For this review, take the finished solid that the model builds, in its own axes (mm). Face numbers are marked on the shaded views. A direction names the side the tool comes from. Round coordinates to 2 decimals unless told otherwise and drop trailing zeros. Write each loop counter-clockwise with the first axis right and the second up, starting at its lowest first coordinate (ties: lowest second). Pieces come first, ordered by that corner, then holes. Notation, with made-up numbers: (23.25, 4.25) -> (61.25, 4.25) arc R34 ccw to (61.25, 41.25) -> close; hole circle Ø7 at (-18, 88). An arc over 180 degrees is marked (long way). Write each question's results on one line, items separated by ' | '. Start each with the question number.
Item 1: Add section D-D (z = 4.5). State the section outline as (x, y) points.
Item 2: Add section C-C (z = 0.75). State the section outline as (x, y) points, plus the area to 3 significant figures.
Item 3: Add section B-B (y = -2.5). State the section outline as (x, z) points.
Item 4: Clearance check with flat-ended pins moving along their axes: pin 1 (0.5 mm diameter, centred on y = -4.5, z = 2.5, fed in from +X); pin 2 (3 mm diameter, centred on x = -3, y = -2, fed in from -Z); pin 3 (3 mm diameter, centred on x = -3.5, y = -3.5, fed in from +Z). State where each tip first meets the part, or that it passes through.
Item 5: The part is to be moulded in two halves that separate along X. For the marked faces 5, 6 and 7, say which applies: +X half, -X half, draft (parallel to the pull), parting line (faces both ways), or undercut.
Item 6: To check wall thickness, follow line 1 along X through (y, z) = (-3, 2.5); line 2 along Y through (x, z) = (19.5, 1); line 3 along X through (y, z) = (-2.5, 3). State the ranges of each line that lie inside material, in increasing order.
Item 7: Add section A-A (x = -4). State the section outline as (y, z) points, plus the area to 3 significant figures.
Item 8: Tool access review of the marked faces 1, 2, 3 and 4: name each direction out of +Z, -Z, +X, -X, +Y, -Y from which nothing blocks a thin tool from reaching the whole face with its end or side.
from build123d import *

# Parameters (mm, degrees)
F1_DEPTH = 6
F2_R     = 1.5
F3_DEPTH = 1.5
F4_R     = 1.5
F4_W     = 1.5
F4_H     = 6
F5_DEPTH = 1.5


with BuildPart() as f1:
    # F0 (on Front) → F1 (new body)
    with BuildSketch(Plane.XZ):
        with BuildLine():
            Line((15, 3), (15, 0))
            Line((15, 0), (16.5, 0))
            Line((16.5, 0), (16.5, 3))
            ThreePointArc((16.5, 3), (15.474874, 5.474874), (13, 6.5))
            Line((13, 6.5), (2, 6.5))
            ThreePointArc((2, 6.5), (-0.474874, 5.474874), (-1.5, 3))
            Line((-1.5, 3), (-1.5, 2))
            Line((-1.5, 2), (0, 2))
            Line((0, 2), (0, 3))
            ThreePointArc((0, 3), (0.585786, 4.414214), (2, 5))
            Line((2, 5), (13, 5))
            ThreePointArc((13, 5), (14.414214, 4.414214), (15, 3))
        make_face()
    extrude(amount=F1_DEPTH)

    # F2 (on Top) → F3 (join)
    with BuildSketch(Plane.XY):
        with BuildLine():
            Line((16.5, 0), (16.5, -6))
            Line((16.5, -6), (19.5, -6))
            ThreePointArc((19.5, -6), (21.62132, -5.12132), (22.5, -3))
            ThreePointArc((22.5, -3), (21.62132, -0.87868), (19.5, 0))
            Line((19.5, 0), (16.5, 0))
        make_face()
        with Locations((19.5, -3)):
            Circle(F2_R, mode=Mode.SUBTRACT)
    extrude(amount=F3_DEPTH)

    # F4 (on face) → F5 (join)
    with BuildSketch(Plane(origin=(0, 0, 2), x_dir=(1, 0, 0), z_dir=(0, 0, -1))):
        with BuildLine():
            Line((-1.5, 6), (-4.5, 6))
            ThreePointArc((-4.5, 6), (-6.62132, 5.12132), (-7.5, 3))
            ThreePointArc((-7.5, 3), (-6.62132, 0.87868), (-4.5, 0))
            Line((-4.5, 0), (-1.5, 0))
            Line((-1.5, 0), (-1.5, 6))
        make_face()
        with Locations((-4.5, 3)):
            Circle(F4_R, mode=Mode.SUBTRACT)
        with Locations((-0.75, 3)):
            Rectangle(F4_W, F4_H)
    extrude(amount=-F5_DEPTH)


solid = f1.part
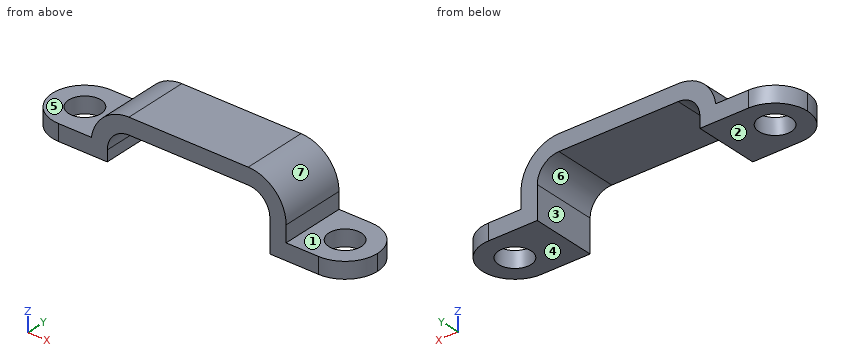
Responses:
1) outline: (-1.16, -6) -> (0.68, -6) -> (0.68, 0) -> (-1.16, 0) -> close; (14.32, -6) -> (16.16, -6) -> (16.16, 0) -> (14.32, 0) -> close
2) outline: (15, -6) -> (19.5, -6) arc R3 ccw to (22.5, -3) arc R3 ccw to (19.5, 0) -> (15, 0) -> close; hole circle Ø3 at (19.5, -3) | area: 34.1 mm^2
3) outline: (-7.46, 2) -> (-5.91, 2) -> (-5.91, 3.5) -> (-7.46, 3.5) -> close; (-3.09, 2) -> (0, 2) -> (0, 3) arc R2 cw to (2, 5) -> (13, 5) arc R2 cw to (15, 3) -> (15, 0) -> (18.09, 0) -> (18.09, 1.5) -> (16.5, 1.5) -> (16.5, 3) arc R3.5 ccw to (13, 6.5) -> (2, 6.5) arc R3.5 ccw to (-1.46, 3.5) -> (-3.09, 3.5) -> close; (20.91, 0) -> (22.46, 0) -> (22.46, 1.5) -> (20.91, 1.5) -> close
4) pin 1: stops at x = 16.5 | pin 2: stops at z = 2 | pin 3: stops at z = 3.5
5) face 5: draft | face 6: undercut | face 7: +X half
6) line 1: x = -7.5 to -6, -3 to 0, 15 to 16.5 | line 2: y = -6 to -4.5, -1.5 to 0 | line 3: x = -7.46 to -5.91, -3.09 to 0, 15 to 16.5
7) outline: (-6, 2) -> (-4.41, 2) -> (-4.41, 3.5) -> (-6, 3.5) -> close; (-1.59, 2) -> (0, 2) -> (0, 3.5) -> (-1.59, 3.5) -> close | area: 4.76 mm^2
8) face 1: +Z, +X, +Y, -Y | face 2: -Z, -X, +Y, -Y | face 3: -Z, +Y, -Y | face 4: -Z, +X, -X, +Y, -Y
